from build123d import *

# Parameters (mm, degrees)
SKETCH_2_R               = 1.5
CUT_EXTRUDE_1_DEPTH      = 11
SKETCH_2_3_R             = 3
SKETCH_2_3_R_2           = 1.5
CUT_EXTRUDE_2_DEPTH      = 3
PATTERN_CIRCULAR_1_COUNT = 10
CHAMFER_1_SIZE           = 2


with BuildPart() as part:
    # Sketch 1 → Revolve 1 (revolve)
    with BuildSketch(Plane.XY):
        Polygon((18.23409983, 96.6), (16.31211603, 96.6), (7.79621586, 88.6), (3.23409983, 88.6), (3.23409983, 96.6), (-13.75, 96.6), (-13.75, 39.865515574), (-16.661143686, 39.865515574), (-16.661143686, 30), (-13.75, 30), (-13.75, 0), (-18.75, 0), (-18.75, 101.69494665), (-18.75, 106.6), (11.163032018, 106.6), (18.23409983, 99.528932188), align=None)
    revolve(axis=Axis((58.23409983, 90.171963423, 0), (0, 1, 0)))

    # Sketch 2 → Cut-Extrude 1 (cut, through all)
    with BuildSketch(Plane.XZ.offset(-96.6)):
        with Locations((58.23409983, 63.75)):
            Circle(SKETCH_2_R)
    cut_extrude_1 = extrude(amount=-CUT_EXTRUDE_1_DEPTH, mode=Mode.SUBTRACT)

    # Sketch 2_3 → Cut-Extrude 2 (cut)
    with BuildSketch(Plane.XZ.offset(-96.6)):
        with Locations((58.23409983, 63.75)):
            Circle(SKETCH_2_3_R)
        with Locations((58.23409983, 63.75)):
            Circle(SKETCH_2_3_R_2, mode=Mode.SUBTRACT)
    cut_extrude_2 = extrude(amount=-CUT_EXTRUDE_2_DEPTH, mode=Mode.SUBTRACT)

    # Pattern Circular 1: Cut-Extrude 1, Cut-Extrude 2 ×10 about axis
    pattern_circular_1_axis = Axis((58.23409983, 0, 0), (0, 1, 0))
    for i in range(1, PATTERN_CIRCULAR_1_COUNT):
        add(cut_extrude_1.rotate(pattern_circular_1_axis, i * 360 / PATTERN_CIRCULAR_1_COUNT), mode=Mode.SUBTRACT)
        add(cut_extrude_2.rotate(pattern_circular_1_axis, i * 360 / PATTERN_CIRCULAR_1_COUNT), mode=Mode.SUBTRACT)

    # Chamfer 1
    chamfer_1_edges = [part.edges().sort_by_distance(p)[0] for p in [
        (135.21819966, 106.6, 0),
    ]]
    chamfer(chamfer_1_edges, length=CHAMFER_1_SIZE)


solid = part.part
Source: CAD feature listing. Evaluate the final solid. Frame: model axes, mm. A direction names the side the tool comes from. Round coordinates to 2 decimals unless told otherwise and drop trailing zeros. Loops run counter-clockwise (first coordinate to the right, second up) from the corner with the lowest first, then second, coordinate; pieces in that order, holes last. Notation, with made-up numbers: M 64.25,1.5 L 91.25,1.5 A18 ccw 91.25,17.5 Z; hole C 27.25,65 d8. An arc over 180 degrees is marked long. Return JSON: item names as keys, results as strings. Group by question number.
1. Section query B-B on y = 32. Output: boundary loops of the cut face in (x, z).
2. Section query D-D on y = 79. Output: boundary loops of the cut face in (x, z).
3. Material intervals for line 1 along Z through (x, y) = (58.5, 13.5); line 2 along Y through (x, z) = (127, -29); line 3 along Y through (x, z) = (127.5, -33.5), sorted ascending. Write a range as from..to.
4. Reachability of faces 4 (the face through (19.754, 99.872, 12.118)), 5 (the face through (19, 39.866, 61)), 6 (the face through (59.62, 98.08, 61.09)) from +Z, -Z, +X, -X, +Y, -Y: full face, straight path, thin tool, end or side. Return the list, or none.
5. Mould query, pull axis X, two halves, no side actions, for faces 1 (the face through (119.33, 51.57, -46.84)), 2 (the face through (60, 99.6, -63)), 3 (the face through (103, 0, -57)). Classes: released by +X, released by -X, zero draft, split by the parting line, or undercut.
6. Pin query (flat end, axial travel): pin 1 (5 mm diameter, centred on x = 66.5, z = 57.5, fed in from -Y); pin 2 (3.5 mm diameter, centred on x = 95.71, z = 51.57, fed in from -Y); pin 3 (2 mm diameter, centred on x = 93, y = 91, fed in from +Z). Return the tip coordinate at first contact, or that it passes through.
7. Section query C-C on y = 91.5. Output: boundary loops of the cut face in (x, z).
Checks:
{
 "1": {"outline": "C 58.23,0 d153.97; hole C 58.23,0 d149.79"},
 "2": {"outline": "C 58.23,0 d153.97; hole C 58.23,0 d143.97"},
 "3": {"line 1": "z = -76.98..-71.98, 71.98..76.98", "line 2": "y = 0..30, 39.87..106.6", "line 3": "y = 0..104.64"},
 "4": {"face 4": "+Y", "face 5": "none", "face 6": "-Y"},
 "5": {"face 1": "split by the parting line", "face 2": "undercut", "face 3": "zero draft"},
 "6": {"pin 1": "stops at y = 96.6", "pin 2": "stops at y = 99.6", "pin 3": "stops at z = 69.18"},
 "7": {"outline": "C 58.23,0 d153.97; C 58.23,0 d110; hole C 58.23,0 d143.97; hole C 58.23,0 d94.7"}
}
